Source: CAD feature listing. Evaluate the final solid. Frame: model axes, mm. Round coordinates to 2 decimals unless told otherwise and drop trailing zeros. Write each loop counter-clockwise with the first axis right and the second up, starting at its lowest first coordinate (ties: lowest second). Pieces come first, ordered by that corner, then holes. Notation, with made-up numbers: M -35.5,38.5 L -1.5,38.5 A26 ccw -1.5,56.5 Z; hole C 49.25,16.25 d2. An arc over 180 degrees is marked long. Put each result on its own line as item: value. Start each with the question number.
Autodesk Inventor part; units mm, degrees
ref_plane "YZ Plane" through (0, 0, 0) normal (1, 0, 0) x (0, 1, 0)
ref_plane "XZ Plane" through (0, 0, 0) normal (0, 1, 0) x (-1, 0, 0)
ref_plane "XY Plane" through (0, 0, 0) normal (0, 0, 1) x (1, 0, 0)
sketch "Sketch1" plane through (0, 0, 0) normal (0, 1, 0) x (-1, 0, 0)
  circle A0 centre (0, 0) radius 203.2
  dimension "d0" = 406.4
extrude "Extrusion1" add sketch "Sketch1" along normal blind 4.7625
sketch "Sketch2" plane through (0, 4.7625, 0) normal (0, 1, 0) x (1, 0, 0)
  point P0 (0, 0)
  point P1 (-88.9, 64)
  point P2 (-176.9, 64)
  point P3 (-88.9, -64)
  point P4 (-176.9, -64)
  dimension "d3" = 0
  dimension "d4" = 0
  dimension "d5" = 0
  dimension "d6" = 0
  dimension "d7" = 128
  dimension "d8" = 88
  dimension "d9" = 64
  dimension "d10" = 88.9
hole "Hole1" at (-88.9, 4.7625, -64) at (-176.9, 4.7625, -64) at (-88.9, 4.7625, 64) at (-176.9, 4.7625, 64) direction (0, -1, 0) diameter 3.2766 end through all
sketch "Sketch3" plane through (0, 4.7625, 0) normal (0, 1, 0) x (1, 0, 0)
  point P0 (0, 0)
  point P1 (88.9, 64)
  point P2 (176.9, 64)
  point P3 (88.9, -62)
  point P4 (176.9, -62)
  dimension "d18" = 0
  dimension "d19" = 0
  dimension "d20" = 0
  dimension "d21" = 0
  dimension "d22" = 126
  dimension "d23" = 88
  dimension "d24" = 64
  dimension "d25" = 88.9
hole "Hole2" at (88.9, 4.7625, -64) at (176.9, 4.7625, -64) at (88.9, 4.7625, 62) at (176.9, 4.7625, 62) direction (0, -1, 0) diameter 3.2766 end through all
sketch "Sketch4" plane through (0, 4.7625, 0) normal (0, 1, 0) x (1, 0, 0)
  point P0 (0, 0)
  point P1 (-38.1, 12.7)
  point P2 (38.1, 12.7)
  dimension "d33" = 38.1
  dimension "d34" = 0
  dimension "d35" = 76.2
  dimension "d125" = 12.7
hole "Hole3" at (-38.1, 4.7625, -12.7) at (38.1, 4.7625, -12.7) direction (0, -1, 0) diameter 5.1054 end through all
sketch "Sketch5" plane through (0, 4.7625, 0) normal (0, 1, 0) x (1, 0, 0)
  line L0 (-79.375, -50.8) -> (79.375, -50.8)
  line L1 (79.375, -50.8) -> (79.375, -418.3154)
  line L2 (79.375, -418.3154) -> (-79.375, -418.3154)
  line L3 (-79.375, -418.3154) -> (-79.375, -50.8)
  point P0 (0, 0)
  dimension "d44" = 158.75
  dimension "d45" = 79.375
  dimension "d46" = 50.8
extrude "Extrusion2" cut sketch "Sketch5" against normal blind 25.4
sketch "Sketch6" plane through (0, 4.7625, 0) normal (0, 1, 0) x (1, 0, 0)
  line L0 (-85.725, -133.35) -> (85.725, -133.35)
  line L1 (85.725, -133.35) -> (85.725, -214.7916)
  line L2 (85.725, -214.7916) -> (-85.725, -214.7916)
  line L3 (-85.725, -214.7916) -> (-85.725, -133.35)
  line L4 (-79.375, -50.8) -> (79.375, -50.8)
  line L5 (-79.375, -187.0557) -> (-79.375, -50.8)
  line L6 (79.375, -50.8) -> (79.375, -187.0557)
  point P0 (0, 0)
  dimension "d49" = 82.55
  dimension "d50" = 6.35
  dimension "d51" = 6.35
extrude "Extrusion3" cut sketch "Sketch6" against normal blind 25.4 contours L0 L1 L2 L3
sketch "Sketch8" plane through (0, 4.7625, 0) normal (0, 1, 0) x (1, 0, 0)
  line L0 (-85.725, -133.35) -> (-79.375, -133.35)
  line L1 (-85.725, -184.2321) -> (-85.725, -133.35)
  point P0 (0, 0)
  point P1 (-136.525, -118.11)
  point P2 (-92.075, -118.11)
  point P3 (-136.525, -137.16)
  point P4 (-92.075, -137.16)
  dimension "d65" = 0
  dimension "d66" = 0
  dimension "d67" = 0
  dimension "d68" = 44.45
  dimension "d69" = 19.05
  dimension "d70" = 0
  dimension "d71" = 15.24
  dimension "d72" = 6.35
hole "Hole5" at (-136.525, 4.7625, 118.11) at (-92.075, 4.7625, 118.11) at (-136.525, 4.7625, 137.16) at (-92.075, 4.7625, 137.16) direction (0, -1, 0) diameter 4.4958 end through all
sketch "Sketch9" plane through (0, 4.7625, 0) normal (0, 1, 0) x (1, 0, 0)
  point P0 (0, 0)
  point P1 (-190.5, 0)
  point P2 (-171.45, 88.9)
  point P3 (-171.45, -88.9)
  dimension "d80" = 190.5
  dimension "d81" = 171.45
  dimension "d82" = 88.9
  dimension "d83" = 88.9
  dimension "d84" = 171.45
hole "Hole6" at (-190.5, 4.7625, 0) at (-171.45, 4.7625, -88.9) at (-171.45, 4.7625, 88.9) direction (0, -1, 0) diameter 4.4958 end through all
sketch "Sketch10" plane through (0, 4.7625, 0) normal (0, 1, 0) x (1, 0, 0)
  point P0 (0, 0)
  point P1 (196.85, 0)
  point P2 (171.45, 88.9)
  point P3 (171.45, -88.9)
  dimension "d92" = 0
  dimension "d93" = 196.85
  dimension "d94" = 171.45
  dimension "d95" = 171.45
  dimension "d96" = 88.9
  dimension "d97" = 88.9
hole "Hole7" at (196.85, 4.7625, 0) at (171.45, 4.7625, -88.9) at (171.45, 4.7625, 88.9) direction (0, -1, 0) diameter 4.4958 end through all
sketch "Sketch11" plane through (0, 4.7625, 0) normal (0, 1, 0) x (1, 0, 0)
  line L0 (-153.6895, -146.05) -> (154.4346, -146.05)
  line L1 (154.4346, -146.05) -> (154.4346, -205.4298)
  line L2 (154.4346, -205.4298) -> (-153.6895, -205.4298)
  line L3 (-153.6895, -205.4298) -> (-153.6895, -146.05)
  line L4 (-79.375, -50.8) -> (79.375, -50.8)
  point P0 (0, 0)
  dimension "d105" = 95.25
extrude "Extrusion4" cut sketch "Sketch11" against normal blind 25.4
sketch "Sketch12" plane through (0, 4.7625, 0) normal (0, 1, 0) x (1, 0, 0)
  point P0 (0, 0)
  point P1 (-76.2, 114.3)
  point P2 (-76.2, -12.7)
  point P3 (76.2, 114.3)
  point P4 (76.2, -12.7)
  dimension "d108" = 0
  dimension "d109" = 0
  dimension "d110" = 0
  dimension "d111" = 0
  dimension "d112" = 76.2
  dimension "d113" = 76.2
  dimension "d115" = 127
  dimension "d123" = 12.7
hole "Hole8" at (-76.2, 4.7625, -114.3) at (-76.2, 4.7625, 12.7) at (76.2, 4.7625, -114.3) at (76.2, 4.7625, 12.7) direction (0, -1, 0) diameter 4.4958 end through all
sketch "Sketch13" plane through (0, 4.7625, 0) normal (0, 1, 0) x (1, 0, 0)
  circle A0 centre (-38.1, 12.7) radius 2.5527
  point P0 (0, 0)
  point P1 (-25.4, 133.35)
  point P2 (25.4, 133.35)
  dimension "d127" = 0
  dimension "d128" = 50.8
  dimension "d129" = 12.7
  dimension "d137" = 120.65
hole "Hole9" at (-25.4, 4.7625, -133.35) at (25.4, 4.7625, -133.35) direction (0, -1, 0) diameter 4.4958 end through all
sketch "Sketch14" plane through (0, 4.7625, 0) normal (0, 1, 0) x (1, 0, 0)
  circle A0 centre (-127, 107.95) radius 19.05
  circle A1 centre (127, 107.95) radius 19.05
  point P0 (0, 0)
  dimension "d138" = 38.1
  dimension "d139" = 127
  dimension "d140" = 107.95
  dimension "d141" = 38.1
  dimension "d142" = 0
  dimension "d143" = 127
extrude "Extrusion5" cut sketch "Sketch14" against normal blind 25.4
sketch "Sketch15" plane through (0, 4.7625, 0) normal (0, 1, 0) x (1, 0, 0)
  arc A0 (141.2786, -146.05) -> (-141.2786, -146.05) centre (0, 0) ccw
  point P0 (101.6, -76.2)
  point P1 (101.6, -95.25)
  point P2 (101.6, -101.6)
  point P3 (101.6, -120.65)
  point P4 (127, -120.65)
  point P5 (127, -101.6)
  point P6 (127, -95.25)
  point P7 (127, -76.2)
  dimension "d146" = 0
  dimension "d147" = 0
  dimension "d148" = 0
  dimension "d149" = 0
  dimension "d150" = 0
  dimension "d151" = 19.05
  dimension "d152" = 19.05
  dimension "d153" = 6.35
  dimension "d154" = 0
  dimension "d155" = 0
  dimension "d156" = 0
  dimension "d157" = 0
  dimension "d158" = 25.4
  dimension "d159" = 0
  dimension "d160" = 101.6
  dimension "d161" = 76.2
hole "Hole10" at (101.6, 4.7625, 76.2) at (101.6, 4.7625, 95.25) at (101.6, 4.7625, 101.6) at (101.6, 4.7625, 120.65) at (127, 4.7625, 120.65) at (127, 4.7625, 101.6) at (127, 4.7625, 95.25) at (127, 4.7625, 76.2) direction (0, -1, 0) diameter 3.81 end through all
sketch "Sketch16" plane through (0, 4.7625, 0) normal (0, 1, 0) x (1, 0, 0)
  point P0 (0, 0)
  point P1 (-60.325, 142.875)
  point P2 (-60.325, 180.975)
  point P3 (60.325, 142.875)
  point P4 (60.325, 180.975)
  dimension "d169" = 38.1
  dimension "d170" = 142.875
  dimension "d171" = 60.325
  dimension "d172" = 0
  dimension "d173" = 0
  dimension "d174" = 0
  dimension "d175" = 0
  dimension "d176" = 60.325
hole "Hole11" at (-60.325, 4.7625, -142.875) at (-60.325, 4.7625, -180.975) at (60.325, 4.7625, -142.875) at (60.325, 4.7625, -180.975) direction (0, -1, 0) diameter 4.4958 end through all
properties part number "TopPlate"
(1) Section query A-A (x = -125). Return loops of the section in (y, z), and give its area (3 significant figures).
(2) Section query C-C (y = 3.5). Count the separate pieces of the cut face and the enclosed holes in it, and give its area (3 significant figures).
(3) Section query B-B (x = 0). Return loops of the section in (y, z).
(4) Contact query for flat-ended pins moving along their axis: P1, Ø4, axis at x = 60.325, z = -142.875, coming from the +Y side; P2, Ø1.4, axis at y = 2, z = 101.5, coming from the +X side; P3, Ø1.5, axis at x = -33.5, y = 4, coming from the -Z side; P4, Ø1, axis at x = -108, y = 1.5, coming from the -Z side. Output: stop coordinate, or through.
(5) Section query D-D (z = -42.5). Return loops of the section in (x, y), and give its area (3 significant figures).
(6) Ray query, line 1 along X through (y, z) = (1, 137.16) (3 decimals); line 2 along X through (y, z) = (1.75, 64) (3 decimals); line 3 along X through (y, z) = (2.55, -118). Return the intervals inside material, ascending.
(7) Pull-direction query (Z, two-part tool) for faces 1 (the cylindrical face through (-6.749, 2.348, -203.088)), 2 (the cylindrical face through (-116.759, 2.415, -124.013)), 3 (the cylindrical face through (137.241, 2.415, -124.013)), 4 (the flat face through (3, 4.762, -26)); classes: +Z half, -Z half, draft (parallel to the pull), parting line (faces both ways), or undercut.
Entries:
1. outline: M 0,-160.2 L 4.76,-160.2 L 4.76,-126.89 L 0,-126.89 Z; M 0,-89.01 L 4.76,-89.01 L 4.76,146.05 L 0,146.05 Z
1. area: 1,280 mm2
2. separate pieces: 1
2. enclosed holes: 40
2. area: 101,000 mm2
3. outline: M 0,-203.2 L 4.76,-203.2 L 4.76,50.8 L 0,50.8 Z
4. P1: through
4. P2: x = 176.44
4. P3: z = -200.54
4. P4: z = -172.44
5. outline: M -198.71,0 L 198.71,0 L 198.71,4.76 L -198.71,4.76 Z
5. area: 1,890 mm2
6. line 1: -149.925 to -138.773, -134.277 to -94.323, -89.827 to -85.725, 85.725 to 149.925
6. line 2: -192.858 to -178.538, -175.262 to -90.538, -87.262 to -79.375, 79.375 to 192.858
6. line 3: -165.43 to -143.18, -110.82 to 110.82, 143.18 to 165.43
7. face 1: parting line
7. face 2: undercut
7. face 3: undercut
7. face 4: draft
